Could you check a few things on this drawing? It's one solid part, dimensions in mm from its lowest x, y, z. Coordinates: 2 decimals unless noted, no trailing zeros. Write each loop counter-clockwise with the first axis right and the second up, starting at its lowest first coordinate (ties: lowest second). Pieces come first, ordered by that corner, then holes. Notation, with made-up numbers: (66, 52.25) - (104, 52.25) arc R30 cw to (104, 75.25) - close; hole circle Ø10 at (67.25, 73). An arc over 180 degrees is marked (long way). Use one line per item in the form item = value. Start each with the question number.
(1) If we section it at C-C on z = 7.75: Please give me the cut outline in (x, y), then the cut area to 3 significant figures.
(2) If we section it at A-A on y = 10: Please give me the cut outline in (x, z).
(3) If we section it at D-D on y = 3.75: Please give me the cut outline in (x, z).
(4) Thinking about a two-plate mould opening in X: for the marked faces 1, 2, 3 and 4, which applies, pulls with the +X half, pulls with the -X half, needs draft (parallel to the pull), parting line crosses it, or undercut?
(5) If I drill on probe 1 along Y at (x, z) = (10, 4); probe 2 along X at (y, z) = (2.5, 2.75); probe 3 along Y at (x, z) = (13.75, 2.25), over which ranges is the centre line in solid material (lowest first)? Write a range as from..to.
(6) For pin 1 Ø6.5 at (x, y) = (10, 10) entering from +Z; pin 2 Ø1.5 at (y, z) = (8.5, 4) entering from -X; pin 3 Ø1.5 at (y, z) = (5.5, 6.5) entering from +X, each with a flat end and sliding along its axis, tell me the tip position at first contact or that it passes through.
(7) If we section it at B-B on x = 10: Please give me the cut outline in (y, z).
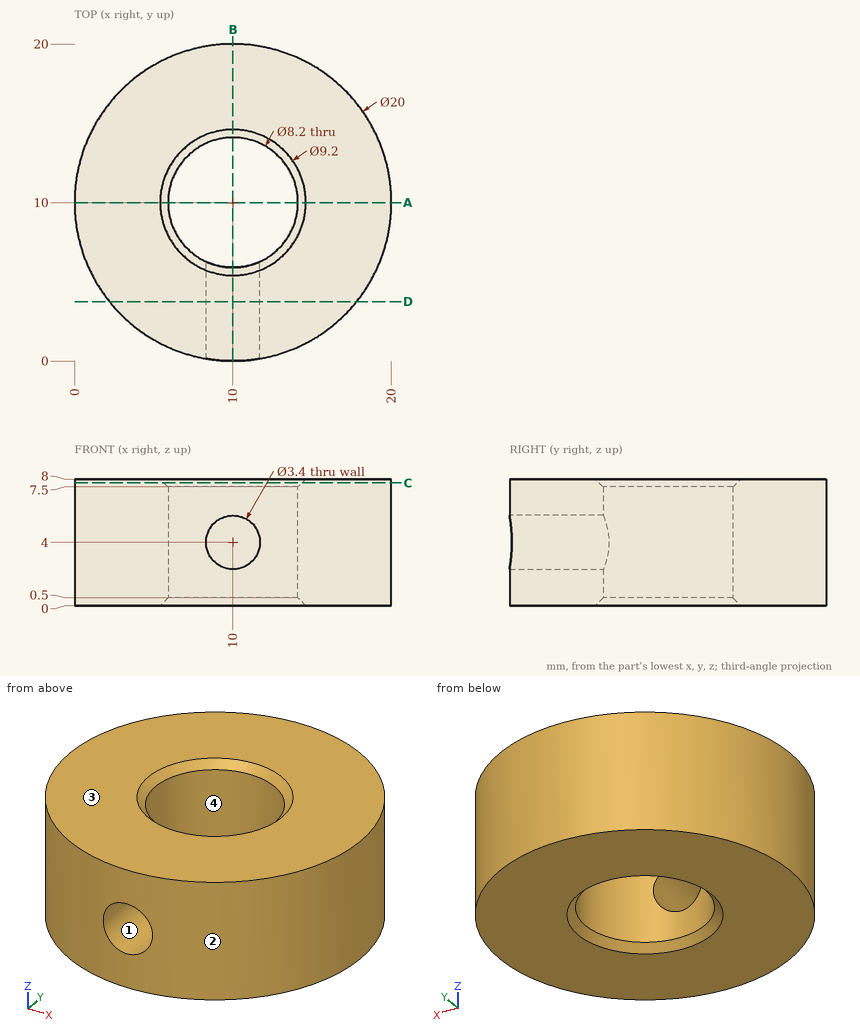
Reported:
q1.outline = circle Ø20 at (10, 10); hole circle Ø8.7 at (10, 10)
q1.area = 255 mm2
q2.outline = (0, 0) - (5.4, 0) - (5.9, 0.5) - (5.9, 7.5) - (5.4, 8) - (0, 8) - close; (14.1, 0.5) - (14.6, 0) - (20, 0) - (20, 8) - (14.6, 8) - (14.1, 7.5) - close
q3.outline = (2.19, 0) - (17.81, 0) - (17.81, 8) - (2.19, 8) - close; hole circle Ø3.4 at (10, 4)
q4.face_1 = undercut
q4.face_2 = parting line crosses it
q4.face_3 = needs draft
q4.face_4 = undercut
q5.probe_1 = 14.1..20
q5.probe_2 = 3.39..8.85, 11.15..16.61
q5.probe_3 = 0.73..8.34, 11.66..19.27
q6.pin_1 = through
q6.pin_2 = 0.03
q6.pin_3 = 19.27
q7.outline = (0, 0) - (5.4, 0) - (5.9, 0.5) - (5.9, 2.3) - (0, 2.3) - close; (0, 5.7) - (5.9, 5.7) - (5.9, 7.5) - (5.4, 8) - (0, 8) - close; (14.1, 0.5) - (14.6, 0) - (20, 0) - (20, 8) - (14.6, 8) - (14.1, 7.5) - close
